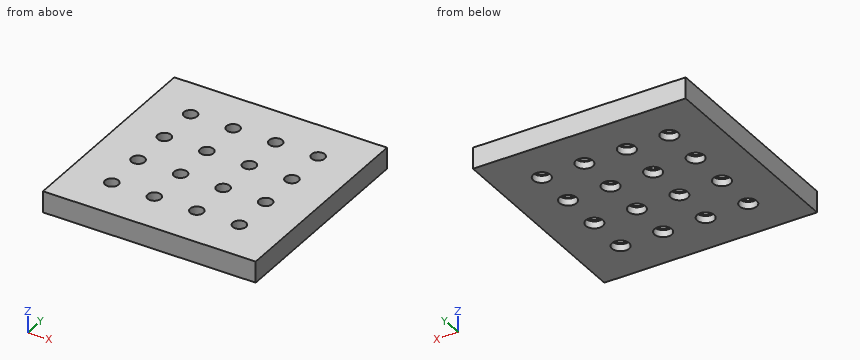
from build123d import *

# Parameters (mm, degrees)
F0_W     = 150
F0_H     = 150
F0_R     = 6.05
F0_R_2   = 4.7
F1_DEPTH = 15
F2_DEPTH = 15
F3_DEPTH = 10
F4_DEPTH = 10
F5_DEPTH = 10
F6_DEPTH = 25
F7_DEPTH = 10


with BuildPart() as f1:
    # F0 (on Top) → F1 (new body)
    with BuildSketch(Plane.XY):
        with Locations((-75, 75)):
            Rectangle(F0_W, F0_H)
        with Locations((-120, 30)):
            Circle(F0_R, mode=Mode.SUBTRACT)
        with Locations((-90, 30)):
            Circle(F0_R, mode=Mode.SUBTRACT)
        with Locations((-120, 60)):
            Circle(F0_R, mode=Mode.SUBTRACT)
        with Locations((-90, 60)):
            Circle(F0_R, mode=Mode.SUBTRACT)
        with Locations((-60, 30)):
            Circle(F0_R, mode=Mode.SUBTRACT)
        with Locations((-30, 30)):
            Circle(F0_R, mode=Mode.SUBTRACT)
        with Locations((-60, 60)):
            Circle(F0_R, mode=Mode.SUBTRACT)
        with Locations((-30, 60)):
            Circle(F0_R, mode=Mode.SUBTRACT)
        with Locations((-120, 90)):
            Circle(F0_R, mode=Mode.SUBTRACT)
        with Locations((-90, 90)):
            Circle(F0_R, mode=Mode.SUBTRACT)
        with Locations((-120, 120)):
            Circle(F0_R, mode=Mode.SUBTRACT)
        with Locations((-90, 120)):
            Circle(F0_R, mode=Mode.SUBTRACT)
        with Locations((-60, 90)):
            Circle(F0_R, mode=Mode.SUBTRACT)
        with Locations((-30, 90)):
            Circle(F0_R, mode=Mode.SUBTRACT)
        with Locations((-60, 120)):
            Circle(F0_R, mode=Mode.SUBTRACT)
        with Locations((-30, 120)):
            Circle(F0_R, mode=Mode.SUBTRACT)
        with Locations((-120, 30)):
            Circle(F0_R)
        with Locations((-120, 30)):
            Circle(F0_R_2, mode=Mode.SUBTRACT)
        with Locations((-120, 30)):
            Circle(F0_R_2)
    extrude(amount=-F1_DEPTH)

    # F0 (on Top) → F2 (cut)
    with BuildSketch(Plane.XY):
        with Locations((-120, 30)):
            Circle(F0_R_2)
    extrude(amount=-F2_DEPTH, mode=Mode.SUBTRACT)

    # F0 (on Top) → F3 (cut)
    with BuildSketch(Plane.XY):
        with Locations((-120, 30)):
            Circle(F0_R)
        with Locations((-120, 30)):
            Circle(F0_R_2, mode=Mode.SUBTRACT)
    extrude(amount=-F3_DEPTH, mode=Mode.SUBTRACT)

    # F0 (on Top) → F4 (join)
    with BuildSketch(Plane.XY):
        with Locations((-120, 60)):
            Circle(F0_R)
        with Locations((-120, 60)):
            Circle(F0_R_2, mode=Mode.SUBTRACT)
        with Locations((-120, 90)):
            Circle(F0_R)
        with Locations((-120, 90)):
            Circle(F0_R_2, mode=Mode.SUBTRACT)
        with Locations((-120, 120)):
            Circle(F0_R)
        with Locations((-120, 120)):
            Circle(F0_R_2, mode=Mode.SUBTRACT)
        with Locations((-90, 120)):
            Circle(F0_R)
        with Locations((-90, 120)):
            Circle(F0_R_2, mode=Mode.SUBTRACT)
        with Locations((-60, 120)):
            Circle(F0_R)
        with Locations((-60, 120)):
            Circle(F0_R_2, mode=Mode.SUBTRACT)
        with Locations((-90, 90)):
            Circle(F0_R)
        with Locations((-90, 90)):
            Circle(F0_R_2, mode=Mode.SUBTRACT)
        with Locations((-90, 60)):
            Circle(F0_R)
        with Locations((-90, 60)):
            Circle(F0_R_2, mode=Mode.SUBTRACT)
        with Locations((-60, 90)):
            Circle(F0_R)
        with Locations((-60, 90)):
            Circle(F0_R_2, mode=Mode.SUBTRACT)
        with Locations((-30, 90)):
            Circle(F0_R)
        with Locations((-30, 90)):
            Circle(F0_R_2, mode=Mode.SUBTRACT)
        with Locations((-30, 60)):
            Circle(F0_R)
        with Locations((-30, 60)):
            Circle(F0_R_2, mode=Mode.SUBTRACT)
        with Locations((-60, 60)):
            Circle(F0_R)
        with Locations((-60, 60)):
            Circle(F0_R_2, mode=Mode.SUBTRACT)
        with Locations((-60, 30)):
            Circle(F0_R)
        with Locations((-60, 30)):
            Circle(F0_R_2, mode=Mode.SUBTRACT)
        with Locations((-90, 30)):
            Circle(F0_R)
        with Locations((-90, 30)):
            Circle(F0_R_2, mode=Mode.SUBTRACT)
        with Locations((-30, 120)):
            Circle(F0_R)
        with Locations((-30, 120)):
            Circle(F0_R_2, mode=Mode.SUBTRACT)
        with Locations((-30, 30)):
            Circle(F0_R)
        with Locations((-30, 30)):
            Circle(F0_R_2, mode=Mode.SUBTRACT)
        with Locations((-120, 30)):
            Circle(F0_R)
        with Locations((-120, 30)):
            Circle(F0_R_2, mode=Mode.SUBTRACT)
    extrude(amount=-F4_DEPTH)

    # F0 (on Top) → F5 (cut)
    with BuildSketch(Plane.XY):
        with Locations((-120, 30)):
            Circle(F0_R)
        with Locations((-120, 30)):
            Circle(F0_R_2, mode=Mode.SUBTRACT)
    extrude(amount=-F5_DEPTH, mode=Mode.SUBTRACT)

    # F0 (on Top) → F6 (cut)
    with BuildSketch(Plane.XY):
        with Locations((-120, 30)):
            Circle(F0_R)
        with Locations((-120, 30)):
            Circle(F0_R_2, mode=Mode.SUBTRACT)
    extrude(amount=-F6_DEPTH, mode=Mode.SUBTRACT)

    # F0 (on Top) → F7 (join)
    with BuildSketch(Plane.XY):
        with Locations((-120, 30)):
            Circle(F0_R)
        with Locations((-120, 30)):
            Circle(F0_R_2, mode=Mode.SUBTRACT)
    extrude(amount=-F7_DEPTH)


solid = f1.part
Work out the finished part from the listing and answer in its coordinate system (mm). Round coordinates to 2 decimals unless told otherwise and drop trailing zeros. Use a Markdown table: item, result.
1) Flat-ended cylindrical pins translate along their axes: pin 1 (6 mm diameter, centred on x = -121.5, y = 122.5, fed in from -Z); pin 2 (8.5 mm diameter, centred on x = -90, y = 30, fed in from -Z). Find the tip coordinate at first contact, or state that the pin passes through.
Taken from the geometry:
| item | result |
|---|---|
| pin 1 | stops at z = -10 |
| pin 2 | passes through |
2) The part is cut by section A-A on z = -2.75. State how many separate pieces and enclosed holes the cut face has, plus the area to 3 significant figures.
Taken from the geometry:
| item | result |
|---|---|
| separate pieces | 1 |
| enclosed holes | 16 |
| area | 21,400 mm2 |
3) Consider line 1 (Y direction, x = -60, z = -8); line 2 (Y direction, x = -30, z = -11.1); line 3 (X direction, y = 59.5, z = -6.25). Determine where each line is inside the solid, lowest interval first. Write a range as [from, to].
Taken from the geometry:
| item | result |
|---|---|
| line 1 | y = [0, 25.3], [34.7, 55.3], [64.7, 85.3], [94.7, 115.3], [124.7, 150] |
| line 2 | y = [0, 23.95], [36.05, 53.95], [66.05, 83.95], [96.05, 113.95], [126.05, 150] |
| line 3 | x = [-150, -124.67], [-115.33, -94.67], [-85.33, -64.67], [-55.33, -34.67], [-25.33, 0] |
